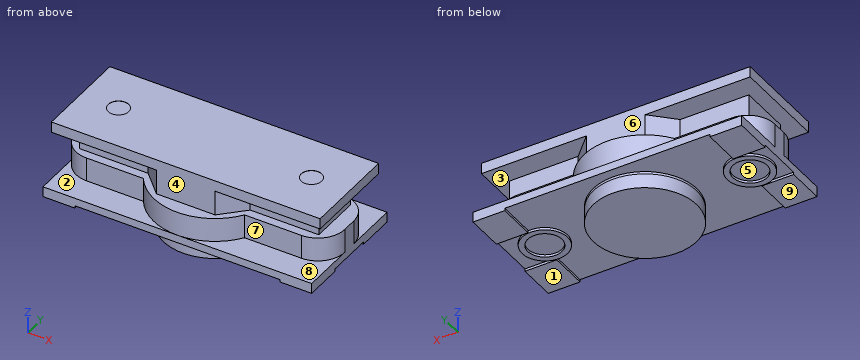
```python
from build123d import *

# Parameters (mm, degrees)
SZKIC1_W                    = 110
SZKIC1_H                    = 50
DODANIE_WYCI_GNI_CIE1_DEPTH = 4.2
SZKIC2_R                    = 21.15
DODANIE_WYCI_GNI_CIE2_DEPTH = 5.9
DODANIE_WYCI_GNI_CIE3_DEPTH = 9.8
ZAOKR_GLENIE1_R             = 11
DODANIE_WYCI_GNI_CIE4_DEPTH = 10.2
SZKIC5_W                    = 110
SZKIC5_H                    = 38.8
DODANIE_WYCI_GNI_CIE5_DEPTH = 4.4
SZKIC6_R                    = 4.2
WYTNIJ_WYCI_GNI_CIE1_DEPTH  = 0.1
SZKIC7_R                    = 9.3
SZKIC7_R_2                  = 7
WYTNIJ_WYCI_GNI_CIE2_DEPTH  = 1


with BuildPart() as part:
    # Szkic1 → Dodanie-wyciągnięcie1 (new body)
    with BuildSketch(Plane.XY):
        Rectangle(SZKIC1_W, SZKIC1_H)
    extrude(amount=DODANIE_WYCI_GNI_CIE1_DEPTH)

    # Szkic2 → Dodanie-wyciągnięcie2 (add)
    with BuildSketch(Plane.XY):
        Circle(SZKIC2_R)
    extrude(amount=-DODANIE_WYCI_GNI_CIE2_DEPTH)

    # Szkic3 → Dodanie-wyciągnięcie3 (add)
    with BuildSketch(Plane.XY.offset(4.2)):
        with BuildLine():
            Line((-55, 14), (-55, -14))
            Line((-55, -14), (-20.712315177, -14))
            ThreePointArc((-20.712315177, -14), (-25, 0), (-20.712315177, 14))
            Line((-20.712315177, 14), (-55, 14))
        make_face()
        with BuildLine():
            ThreePointArc((-20.712315177, 14), (-25, 0), (-20.712315177, -14))
            Line((-20.712315177, -14), (20.712315177, -14))
            ThreePointArc((20.712315177, -14), (23.904056972, -7.32093302), (25, 0))
            ThreePointArc((25, 0), (23.904056972, 7.32093302), (20.712315177, 14))
            Line((20.712315177, 14), (-20.712315177, 14))
        make_face()
        with BuildLine():
            ThreePointArc((20.712315177, 14), (0, 25), (-20.712315177, 14))
            Line((-20.712315177, 14), (20.712315177, 14))
        make_face()
        with BuildLine():
            ThreePointArc((25, 0), (23.904056972, -7.32093302), (20.712315177, -14))
            Line((20.712315177, -14), (55, -14))
            Line((55, -14), (55, 14))
            Line((55, 14), (20.712315177, 14))
            ThreePointArc((20.712315177, 14), (23.904056972, 7.32093302), (25, 0))
        make_face()
        with BuildLine():
            Line((20.712315177, -14), (-20.712315177, -14))
            ThreePointArc((-20.712315177, -14), (0, -25), (20.712315177, -14))
        make_face()
    extrude(amount=DODANIE_WYCI_GNI_CIE3_DEPTH)

    # Zaokrąglenie1
    zaokr_glenie1_edges = [part.edges().sort_by_distance(p)[0] for p in [
        (-55, -14, 9.1),
        (55, -14, 9.1),
        (55, 14, 9.1),
        (-55, 14, 9.1),
    ]]
    fillet(zaokr_glenie1_edges, radius=ZAOKR_GLENIE1_R)

    # Szkic4 → Dodanie-wyciągnięcie4 (add)
    with BuildSketch(Plane.XY.offset(14)):
        Polygon((12, 19.4), (20.9, 10.5), (49, 10.5), (49, -10.5), (20.9, -10.5), (12, -19.4), (-12, -19.4), (-20.9, -10.5), (-49, -10.5), (-49, 10.5), (-20.9, 10.5), (-12, 19.4), align=None)
    extrude(amount=DODANIE_WYCI_GNI_CIE4_DEPTH)

    # Szkic5 → Dodanie-wyciągnięcie5 (add)
    with BuildSketch(Plane.XY.offset(24.2)):
        Rectangle(SZKIC5_W, SZKIC5_H)
    extrude(amount=DODANIE_WYCI_GNI_CIE5_DEPTH)

    # Szkic6 → Wytnij-wyciągnięcie1 (cut)
    with BuildSketch(Plane.XY.offset(28.6)):
        with Locations((-39.5, 0)):
            Circle(SZKIC6_R)
        with Locations((39.5, 0)):
            Circle(SZKIC6_R)
    extrude(amount=-WYTNIJ_WYCI_GNI_CIE1_DEPTH, mode=Mode.SUBTRACT)

    # Szkic7 → Wytnij-wyciągnięcie2 (cut)
    with BuildSketch(Plane(origin=(0, 0, 0), x_dir=(-1, 0, 0), z_dir=(0, 0, -1))):
        Polygon((42, 9.5), (42, 25), (-42, 25), (-42, 9.5), (-55, 9.5), (-55, -9.5), (-42, -9.5), (-42, -25), (42, -25), (42, -9.5), (55, -9.5), (55, 9.5), align=None)
        with Locations((-41, 0)):
            Circle(SZKIC7_R, mode=Mode.SUBTRACT)
        with BuildLine():
            ThreePointArc((21.15, 0), (0, -21.15), (-21.15, 0))
            ThreePointArc((-21.15, 0), (0, 21.15), (21.15, 0))
        make_face(mode=Mode.SUBTRACT)
        with Locations((43, 0)):
            Circle(SZKIC7_R, mode=Mode.SUBTRACT)
        with Locations((43, 0)):
            Circle(SZKIC7_R_2)
        with Locations((-41, 0)):
            Circle(SZKIC7_R_2)
    extrude(amount=-WYTNIJ_WYCI_GNI_CIE2_DEPTH, mode=Mode.SUBTRACT)


solid = part.part
```
Source: CAD feature listing. Evaluate the final solid. Frame: model axes, mm. Face numbers are marked on the shaded views. A direction names the side the tool comes from. Give positions to 0.01 mm unless a question says otherwise; leave off trailing zeros. Loops run counter-clockwise (first coordinate to the right, second up) from the corner with the lowest first, then second, coordinate; pieces in that order, holes last. Notation, with made-up numbers: M 12,7 L 47,7 A6 ccw 47,15 Z; hole C -32.5,35 d10. An arc over 180 degrees is marked long. Put each result on its own line as item: value.
Q1. Mould query, pull axis Z, two halves, no side actions, for the marked faces 6, 7, 8 and 9. Classes: released by +Z, released by -Z, zero draft, split by the parting line, or undercut.
Response values:
face 6: zero draft
face 7: undercut
face 8: undercut
face 9: released by -Z
Q2. Section D-D (x = -8). Return the cut outline in (y, z), and give its area (3 significant figures).
Response values:
outline: M -25,1 L -19.58,1 L -19.58,-5.9 L 19.58,-5.9 L 19.58,1 L 25,1 L 25,4.2 L 23.69,4.2 L 23.69,14 L 19.4,14 L 19.4,28.6 L -19.4,28.6 L -19.4,14 L -23.69,14 L -23.69,4.2 L -25,4.2 Z
area: 1,460 mm²
Q3. Line query: probe 1 along Z at (x, y) = (-31, 14.5); probe 2 along Z at (x, y) = (25, 11.5); probe 3 along Z at (x, y) = (-39.5, -1.5). Output: solid intervals per line, ascending. Write a range as [from, to].
Response values:
probe 1: z = [1, 4.2], [24.2, 28.6]
probe 2: z = [1, 14], [24.2, 28.6]
probe 3: z = [1, 28.5]
Q4. Pin query (flat end, axial travel): P1, Ø1.5, axis at x = 16.5, z = 12.5, coming from the -Y side; P2, Ø15.5, axis at x = -46.5, y = 1.5, coming from the -Z side; P3, Ø2.5, axis at x = 39, y = -1.5, coming from the +Z side. Return the tip coordinate at first contact, or that it passes through.
Response values:
P1: stops at y = -19.41
P2: stops at z = 0
P3: stops at z = 28.5
Q5. Section A-A (x = 28). Return the cut outline in (y, z).
Response values:
outline: M -25,1 L 25,1 L 25,4.2 L 14,4.2 L 14,14 L 10.5,14 L 10.5,24.2 L 19.4,24.2 L 19.4,28.6 L -19.4,28.6 L -19.4,24.2 L -10.5,24.2 L -10.5,14 L -14,14 L -14,4.2 L -25,4.2 Z
Q6. Section C-C (z = 25.5). Return the cut outline in (x, y), and give its area (3 significant figures).
Response values:
outline: M -55,-19.4 L 55,-19.4 L 55,19.4 L -55,19.4 Z
area: 4,270 mm²
Q7. Section B-B (y = -16.5). Return the cut outline in (x, z), and give its area (3 significant figures).
Response values:
outline: M -55,0 L -42,0 L -42,1 L -13.23,1 L -13.23,-5.9 L 13.23,-5.9 L 13.23,1 L 42,1 L 42,0 L 55,0 L 55,4.2 L 18.78,4.2 L 18.78,14 L 14.9,14 L 14.9,24.2 L 55,24.2 L 55,28.6 L -55,28.6 L -55,24.2 L -14.9,24.2 L -14.9,14 L -18.78,14 L -18.78,4.2 L -55,4.2 Z
area: 1,720 mm²
Q8. Reachability of the marked faces 1, 2, 3, 4 and 5 from +Z, -Z, +X, -X, +Y, -Y: full face, straight path, thin tool, end or side. Return the list, or none.
Response values:
face 1: -Z, +X, +Y, -Y
face 2: -X, -Y
face 3: +X
face 4: +Z, +X, -X, -Y
face 5: -Z
